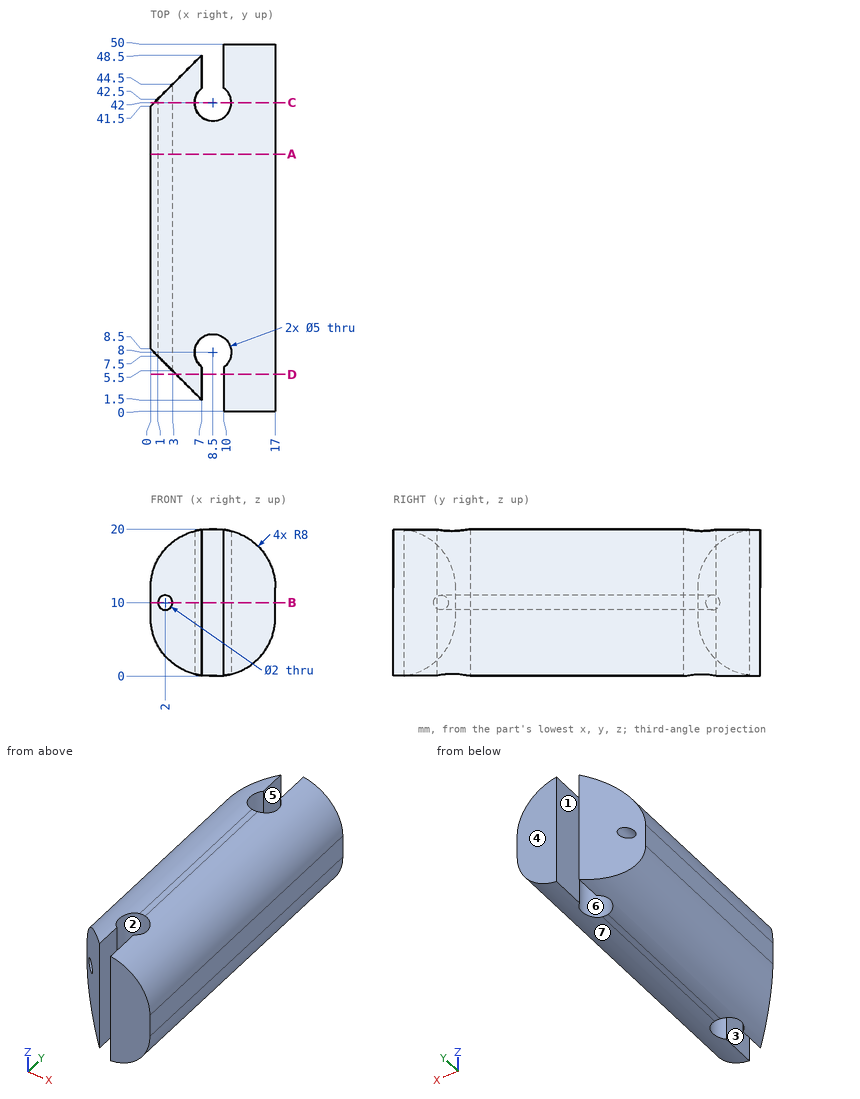
Input: dimensioned drawing with shaded views. Units: mm. Origin: part minimum x, y, z. A direction names the side the tool comes from. Coordinates: 2 decimals unless noted, no trailing zeros. Order: outer loops, then holes, each group sorted by start corner. A loop starts at its lowest first (then second) coordinate and runs counter-clockwise, first axis right, second up.
Item 1: Draft query along X for the marked faces 4, 5, 6 and 7. Return one class per face: released by +X, released by -X, zero draft, split by the parting line, or undercut.
Answer:
face 4: zero draft
face 5: undercut
face 6: undercut
face 7: released by +X
Item 2: Section query B-B (z = 10). Output: boundary loops of the cut face in (x, y), then the cut area to 3 significant figures.
Answer:
outline: (0, 8.5) - (1, 7.5) - (1, 42.5) - (0, 41.5) - close; (3, 5.5) - (7, 1.5) - (7, 6) arc R2.5 cw (long way) to (10, 6) - (10, 0) - (17, 0) - (17, 50) - (10, 50) - (10, 44) arc R2.5 cw (long way) to (7, 44) - (7, 48.5) - (3, 44.5) - close
area: 633 mm2
Item 3: Section query D-D (y = 5). Output: boundary loops of the cut face in (x, z).
Answer:
outline: (3.5, 1.39) arc R8 ccw to (7, 0.06) - (7, 19.94) arc R8 ccw to (3.5, 18.61) - close; (10, 0.06) arc R8 ccw to (17, 8) - (17, 12) arc R8 ccw to (10, 19.94) - close
Item 4: Contact query for flat-ended pins moving along their axis: P1, Ø6.5, axis at y = 45.5, z = 10, coming from the -X side; P2, Ø3, axis at x = 2, z = 10, coming from the +Y side; P3, Ø8, axis at y = 34.5, z = 6, coming from the -X side; P4, Ø2, axis at y = 10.5, z = 2, coming from the -X side (3 decimals). Output: stop coordinate, or through.
Answer:
P1: stops at x = 0.75
P2: stops at y = 45
P3: stops at x = 0
P4: stops at x = 1.755
Item 5: Material intervals for line 1 along X through (y, z) = (5.5, 8.5); line 2 along X through (y, z) = (42, 9.5); line 3 along Y through (x, z) = (10.5, 8.5), sorted ascending.
Answer:
line 1: x = 3 to 7, 10 to 17
line 2: x = 0.5 to 1.13, 2.87 to 6, 11 to 17
line 3: y = 0 to 6.5, 9.5 to 40.5, 43.5 to 50
Item 6: Access query for the marked faces 1, 2 and 3. Directions: +Z, -Z, +X, -X, +Y, -Y. A direction counts if a zero-diameter tool reaches every point of the face in a straight line with its end or side. Return the directions, or none.
Answer:
face 1: +Z, -Z, +Y
face 2: +Z, -Z
face 3: +Z, -Z, -Y
Item 7: Section query A-A (y = 35). Output: boundary loops of the cut face in (x, z).
Answer:
outline: (0, 8) arc R8 ccw to (8, 0) - (9, 0) arc R8 ccw to (17, 8) - (17, 12) arc R8 ccw to (9, 20) - (8, 20) arc R8 ccw to (0, 12) - close; hole circle Ø2 at (2, 10)
Item 8: Section query C-C (y = 42). Output: boundary loops of the cut face in (x, z), then the cut area to 3 significant figures.
Answer:
outline: (0.5, 5.22) arc R8 ccw to (6, 0.25) - (6, 19.75) arc R8 ccw to (0.5, 14.78) - close; (11, 0.25) arc R8 ccw to (17, 8) - (17, 12) arc R8 ccw to (11, 19.75) - close; hole circle Ø2 at (2, 10)
area: 179 mm2
